Design review of the part built by this model. Coordinates are the model's own, in mm. Face numbers are marked on the shaded views. A direction names the side the tool comes from. Coordinates: 2 decimals unless noted, no trailing zeros. Loops run counter-clockwise (first coordinate to the right, second up) from the corner with the lowest first, then second, coordinate; pieces in that order, holes last. Notation, with made-up numbers: M 9,84 L 14,84 A16 ccw 14,93 Z; hole C -24,28.5 d6. An arc over 180 degrees is marked long. Answer as a JSON object with one key per item and string values. Group by question number.
1. Machinability: for the marked faces 4 and 5, which of the approach directions +Z, -Z, +X, -X, +Y, -Y give a long, thin tool a straight path to every point of the face, cutting with its end or side? Answer none if there is none.
2. Consider section A-A (y = 0). State the section outline as (x, z) points, then the cut area to 3 significant figures.
3. To check wall thickness, follow probe 1 along Z at (x, y) = (-7, 0); probe 2 along Y at (x, z) = (-2, 80); probe 3 along Y at (x, z) = (9, -65). State the ranges of each line that lie inside material, in increasing order.
4. Consider section D-D (z = 0). State the section outline as (x, y) points, then the cut area to 3 significant figures.
5. Consider section B-B (z = 130.5). State the section outline as (x, y) points, then the cut area to 3 significant figures.
6. Consider section C-C (x = -0.5). State the section outline as (y, z) points.
7. Insertion check: pin 1 (18 mm diameter, centred on y = 0, z = 0, fed in from -X) (3 decimals); pin 2 (12.5 mm diameter, centred on x = 4, z = 44, fed in from -Y); pin 3 (5 mm diameter, centred on x = -6, y = -77.5, fed in from -Z); pin 4 (5 mm diameter, centred on x = -3.5, y = -76, fed in from +Z). Each pin has a flat end and moves straight along its axis. Give the tip position at first contact, or say it passes through.
8. Draft analysis for pull direction Z (two halves, no side actions). For the marked faces 1, 2 and 3, state which applies: +Z half, -Z half, draft (parallel to the pull), parting line (faces both ways), or undercut.
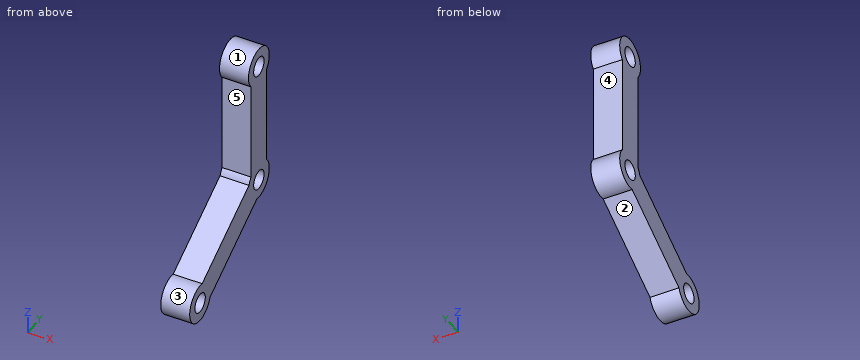
from build123d import *

# Parameters (mm, degrees)
SKETCH2_W           = 30
SKETCH2_H           = 30
SKETCH2_W_2         = 25
SKETCH2_H_2         = 25
SKETCH3_R           = 20
BOSS_EXTRUDE2_DEPTH = 30
SKETCH4_R           = 10
CUT_EXTRUDE1_DEPTH  = 30


with BuildPart() as part:
    # Sweep1: sweep along a path in Sketch1
    with BuildLine(Plane(origin=(0, 0, 0), x_dir=(0, 0, -1), z_dir=(1, 0, 0))) as sweep1_path:
        Line((-130.5, 0), (0, 0))
        Line((0, 0), (65.25, -113.016315194))
    # Sketch2 → Sweep1 (sweep)
    with BuildSketch(Plane.XY.offset(130.5)):
        Rectangle(SKETCH2_W, SKETCH2_H)
        Rectangle(SKETCH2_W_2, SKETCH2_H_2, mode=Mode.SUBTRACT)
    sweep(path=sweep1_path.line, transition=Transition.RIGHT)

    # Sketch3 → Boss-Extrude2 (add)
    with BuildSketch(Plane(origin=(15, 0, 0), x_dir=(0, 0, -1), z_dir=(1, 0, 0))):
        Circle(SKETCH3_R)
        with Locations((65.25, -113.016315194)):
            Circle(SKETCH3_R)
        with Locations((-130.5, 0)):
            Circle(SKETCH3_R)
    extrude(amount=-BOSS_EXTRUDE2_DEPTH)

    # Sketch4 → Cut-Extrude1 (cut)
    with BuildSketch(Plane(origin=(15, 0, 0), x_dir=(0, 0, -1), z_dir=(1, 0, 0))):
        with Locations(Location((-130.5, 0, 0), (0, 0, 90))):
            Circle(SKETCH4_R)
        with Locations(Location((0, 0, 0), (0, 0, 90))):
            Circle(SKETCH4_R)
        with Locations(Location((65.25, -113.016315194, 0), (0, 0, 90))):
            Circle(SKETCH4_R)
    extrude(amount=-CUT_EXTRUDE1_DEPTH, mode=Mode.SUBTRACT)


solid = part.part
Findings below:
{
 "1": {"face 4": "+X, -X, +Y", "face 5": "+X, -X, -Y"},
 "2": {"outline": "M -15,-20 L 15,-20 L 15,-10 L -15,-10 Z; M -15,10 L 15,10 L 15,120.5 L -15,120.5 Z; M -15,140.5 L 15,140.5 L 15,150.5 L -15,150.5 Z; hole M -12.5,20 L 12.5,20 L 12.5,110.5 L -12.5,110.5 Z", "area": "1,650 mm^2"},
 "3": {"probe 1": "z = -20 to -10, 10 to 20, 110.5 to 120.5, 140.5 to 150.5", "probe 2": "y = -15 to -12.5, 12.5 to 15", "probe 3": "y = -133.01 to -123.01, -103.02 to -93.02, -87.58 to -82.58"},
 "4": {"outline": "M -15,-30 L 15,-30 L 15,-10 L -15,-10 Z; M -15,10 L 15,10 L 15,20 L -15,20 Z; hole M -12.5,-25 L 12.5,-25 L 12.5,-20 L -12.5,-20 Z", "area": "775 mm^2"},
 "5": {"outline": "M -15,-20 L 15,-20 L 15,-10 L -15,-10 Z; M -15,10 L 15,10 L 15,20 L -15,20 Z", "area": "600 mm^2"},
 "6": {"outline": "M -109.06,-45.65 A20 ccw long -94.06,-71.63 L -3.96,-19.6 A20 ccw 15,13.23 L 15,117.27 A20 ccw long -15,117.27 L -15,13.23 A20 ccw -18.96,6.38 Z; hole C -113.02,-65.25 d20; hole M -105.75,-46.62 A20 cw -93.25,-68.27 L -7.27,-18.63 A20 cw -19.77,3.02 Z; hole M -12.5,15.61 A20 cw 12.5,15.61 L 12.5,114.89 A20 cw -12.5,114.89 Z; hole C 0,0 d20; hole C 0,130.5 d20"},
 "7": {"pin 1": "passes through", "pin 2": "stops at y = -15", "pin 3": "stops at z = -63.51", "pin 4": "stops at z = -25.11"},
 "8": {"face 1": "undercut", "face 2": "-Z half", "face 3": "parting line"}
}
